Build history of the part. All positions in model axes, mm. Round coordinates to 2 decimals unless told otherwise and drop trailing zeros. Order: outer loops, then holes, each group sorted by start corner. A loop starts at its lowest first (then second) coordinate and runs counter-clockwise, first axis right, second up. Notation, with made-up numbers: M 10,16 L 21,16 A19 cw 21,25 Z; hole C 59.5,82 d9. An arc over 180 degrees is marked long. Use CSV: the item, a comma, the result in double quotes.
from build123d import *

# Parameters (mm, degrees)
SKETCH_1_R      = 1.3
EXTRUDE_1_DEPTH = 3


with BuildPart() as part:
    # 草图1 → 凸台-拉伸1 (new body)
    with BuildSketch(Plane(origin=(0, 0, 0), x_dir=(1, 0, 0), z_dir=(0, 1, 0))):
        Polygon((-65.303381521, 7.5), (-65.303381521, -7.5), (-56, -7.5), (-20, -7.5), (0, -7.5), (25, -7.5), (25, 0), (25, 7.5), (0, 7.5), align=None)
        with Locations((-56, 0)):
            Circle(SKETCH_1_R, mode=Mode.SUBTRACT)
        with Locations((-20, 0)):
            Circle(SKETCH_1_R, mode=Mode.SUBTRACT)
        Circle(SKETCH_1_R, mode=Mode.SUBTRACT)
        with Locations((22.3, 0)):
            Circle(SKETCH_1_R, mode=Mode.SUBTRACT)
    extrude(amount=EXTRUDE_1_DEPTH)


solid = part.part
(1) Drop a flat-ended pin along its axis: pin 1 (2.5 mm diameter, centred on x = -56, z = 0, fed in from +Y). Give the stop position or say it passes through.
Answer block:
pin 1,"passes through"
(2) Cut at B-B, the plane y = 0.8. Give the cut face in (x, z), and give its area (3 significant figures).
Answer block:
outline,"M -65.3,-7.5 L 25,-7.5 L 25,7.5 L -65.3,7.5 Z; hole C -56,0 d2.6; hole C -20,0 d2.6; hole C 0,0 d2.6; hole C 22.3,0 d2.6"
area,"1,330 mm²"
(3) Two-plate mould, pull along X, no slides. Class faces 1 (the face through (-0.17, 1.48, -1.29)), 2 (the face through (-21, 0, -2)), 3 (the face through (25, 1, 0)): released by +X, released by -X, zero draft, split by the parting line, or undercut.
Answer block:
face 1,"undercut"
face 2,"zero draft"
face 3,"released by +X"
(4) Cut at A-A, the plane x = -20. Give the cut face in (y, z).
Answer block:
outline,"M 0,-7.5 L 3,-7.5 L 3,-1.3 L 0,-1.3 Z; M 0,1.3 L 3,1.3 L 3,7.5 L 0,7.5 Z"
(5) Wall check: line 1 (X direction, y = 0.8, z = 0); line 2 (Z direction, x = 22.3, y = 1.05). Give the ranges that are in metal, low to high. Write a range as from..to.
Answer block:
line 1,"x = -65.3..-57.3, -54.7..-21.3, -18.7..-1.3, 1.3..21, 23.6..25"
line 2,"z = -7.5..-1.3, 1.3..7.5"
